Autodesk Inventor part; units mm, degrees
ref_plane "YZ Plane" through (0, 0, 0) normal (1, 0, 0) x (0, 1, 0)
ref_plane "XZ Plane" through (0, 0, 0) normal (0, 1, 0) x (-1, 0, 0)
ref_plane "XY Plane" through (0, 0, 0) normal (0, 0, 1) x (1, 0, 0)
sketch "Sketch1" plane through (0, 0, 0) normal (0, 0, 1) x (1, 0, 0)
  line L0 (0, 37.7) -> (0, -2.9)
  line L1 (-79.8, 0) -> (106.4, 0)
  line L2 (-66.5, 0) -> (66.5, 0)
  line L3 (66.5, 0) -> (66.5, 29)
  line L4 (66.5, 29) -> (-66.5, 29)
  line L5 (-66.5, 29) -> (-66.5, 0)
  dimension "d0" = 133
  dimension "d1" = 29
extrude "Extrusion1" add sketch "Sketch1" along normal blind 1
decal "Decal1"
decal "Decal2"
sketch "Sketch5" plane through (0, 0, 1) normal (0, 0, 1) x (1, 0, 0)
  line L0 (-66.5, 0) -> (-66.5, 29)
  line L1 (66.5, 29) -> (66.5, 0)
  line L2 (-66.5, 19.147) -> (-65.5825, 19.147)
  line L3 (-65.5825, 19.147) -> (-65.5825, 15.2864)
  line L4 (-65.5825, 15.2864) -> (-66.5, 15.2864)
  line L5 (-66.5, 15.2864) -> (-66.5, 19.147)
  line L6 (-66.5, 11.2859) -> (-65.5825, 11.2859)
  line L7 (-65.5825, 11.2859) -> (-65.5825, 7.4252)
  line L8 (-65.5825, 7.4252) -> (-66.5, 7.4252)
  line L9 (-66.5, 7.4252) -> (-66.5, 11.2859)
  circle A0 centre (-65.5825, 17.2167) radius 1.9303
  circle A1 centre (-65.5825, 9.3555) radius 1.9303
  line L10 (66.5, 19.4238) -> (65.1393, 19.4238)
  line L11 (65.1393, 19.4238) -> (65.1393, 15.6247)
  line L12 (65.1393, 15.6247) -> (66.5, 15.6247)
  line L13 (66.5, 15.6247) -> (66.5, 19.4238)
  line L14 (66.5, 11.6256) -> (65.3393, 11.6256)
  line L15 (65.3393, 11.6256) -> (65.3393, 7.8264)
  line L16 (65.3393, 7.8264) -> (66.5, 7.8264)
  line L17 (66.5, 7.8264) -> (66.5, 11.6256)
  circle A2 centre (65.1393, 17.5243) radius 1.8996
  circle A3 centre (65.3393, 9.726) radius 1.8996
  circle A4 centre (-64.4646, 1.8448) radius 1.5
  circle A5 centre (64.8231, 1.8448) radius 1.5
  dimension "d12" = 3
extrude "Extrusion2" cut sketch "Sketch5" against normal through all
sketch "Sketch6" plane through (0, 0, 1) normal (0, 0, 1) x (1, 0, 0)
  line L0 (66.5, 0) -> (-66.5, 0)
  line L1 (3.433, 2.75) -> (4.933, 2.75)
  line L2 (4.933, 2.75) -> (4.933, 0)
  line L3 (4.933, 0) -> (3.433, 0)
  line L4 (3.433, 0) -> (3.433, 2.75)
  circle A0 centre (4.183, 2.75) radius 0.75
  dimension "d15" = 1.5
  dimension "d16" = 2.75
extrude "Extrusion3" cut sketch "Sketch6" against normal through all
sketch "Sketch7" plane through (0, 0, 1) normal (0, 0, 1) x (1, 0, 0)
  line L0 (-46.1031, 8.3659) -> (-58.1031, 8.3659)
  line L1 (-58.1031, 8.3659) -> (-58.1031, 22.3659)
  line L2 (-58.1031, 22.3659) -> (-46.1031, 22.3659)
  line L3 (-46.1031, 22.3659) -> (-46.1031, 8.3659)
  line L4 (-36.7296, 22.3659) -> (-24.7296, 22.3659)
  line L5 (-24.7296, 22.3659) -> (-24.7296, 8.3659)
  line L6 (-24.7296, 8.3659) -> (-36.7296, 8.3659)
  line L7 (-36.7296, 8.3659) -> (-36.7296, 22.3659)
  line L8 (22.9991, 22.3659) -> (34.9991, 22.3659)
  line L9 (34.9991, 22.3659) -> (34.9991, 8.3659)
  line L10 (34.9991, 8.3659) -> (22.9991, 8.3659)
  line L11 (22.9991, 8.3659) -> (22.9991, 22.3659)
  line L12 (40.9859, 22.3659) -> (52.9859, 22.3659)
  line L13 (52.9859, 22.3659) -> (52.9859, 8.3659)
  line L14 (52.9859, 8.3659) -> (40.9859, 8.3659)
  line L15 (40.9859, 8.3659) -> (40.9859, 22.3659)
  dimension "d21" = 14
  dimension "d22" = 12
extrude "Extrusion4" add sketch "Sketch7" along normal blind 0.5
sketch "Sketch8" plane through (0, 0, 0) normal (0, 0, -1) x (-1, 0, 0)
  line L0 (-58.0858, 22.4822) -> (-46.5858, 22.4822)
  line L1 (-46.5858, 22.4822) -> (-46.5858, 8.4822)
  line L2 (-46.5858, 8.4822) -> (-58.0858, 8.4822)
  line L3 (-58.0858, 8.4822) -> (-58.0858, 22.4822)
  line L4 (-36.8395, 22.4822) -> (-25.3395, 22.4822)
  line L5 (-25.3395, 22.4822) -> (-25.3395, 8.4822)
  line L6 (-25.3395, 8.4822) -> (-36.8395, 8.4822)
  line L7 (-36.8395, 8.4822) -> (-36.8395, 22.4822)
  line L8 (23.4032, 22.2455) -> (34.9032, 22.2455)
  line L9 (34.9032, 22.2455) -> (34.9032, 8.4822)
  line L10 (34.9032, 8.4822) -> (23.4032, 8.4822)
  line L11 (23.4032, 8.4822) -> (23.4032, 22.2455)
  line L12 (41.476, 22.1379) -> (52.976, 22.1379)
  line L13 (52.976, 22.1379) -> (52.976, 8.4822)
  line L14 (52.976, 8.4822) -> (41.476, 8.4822)
  line L15 (41.476, 8.4822) -> (41.476, 22.1379)
  dimension "d28" = 11.5
  dimension "d29" = 14
extrude "Extrusion5" add sketch "Sketch8" along normal blind 0.5
sketch "Sketch3" plane through (0, 0, 1) normal (0, 0, 1) x (1, 0, 0)
  line L0 (-66.5, 29) -> (66.5, 29) construction
  line L1 (66.5, 29) -> (66.5, -0.391) construction
  line L2 (66.5, -0.391) -> (-66.5, -0.391) construction
  line L3 (-66.5, -0.391) -> (-66.5, 29) construction
sketch "Sketch4" plane through (0, 0, 0) normal (0, 0, -1) x (-1, 0, 0)
  line L0 (-66.5, 29) -> (66.5, 29) construction
  line L1 (66.5, 29) -> (66.5, -0.391) construction
  line L2 (66.5, -0.391) -> (-66.5, -0.391) construction
  line L3 (-66.5, -0.391) -> (-66.5, 29) construction
properties part number "config - ram"
The listing builds one solid part. Answer for the finished solid, in the listing's coordinates (mm). Coordinates: 2 decimals unless noted, no trailing zeros. Loops run counter-clockwise (first coordinate to the right, second up) from the corner with the lowest first, then second, coordinate; pieces in that order, holes last. Notation, with made-up numbers: M 41.5,70.5 L 66.5,70.5 A24 ccw 66.5,81.5 Z; hole C 51.25,-23 d7. An arc over 180 degrees is marked long. Answer in a Markdown table with one row per item.
1) Find the intervals of material crossed by probe 1 along X at (y, z) = (10.75, 1.2); probe 2 along X at (y, z) = (17.5, -0.1); probe 3 along Y at (x, z) = (28, 1.2), in increasing order.
Answers below:
| item | result |
|---|---|
| probe 1 | -58.1 to -46.1, -36.73 to -24.73, 23 to 35, 40.99 to 52.99 |
| probe 2 | -52.98 to -41.48, -34.9 to -23.4, 25.34 to 36.84, 46.59 to 58.09 |
| probe 3 | 8.37 to 22.37 |
2) Determine the mould class of faces 1 (the cylindrical face through (63.325, 1.911, 0.507)), 2 (the flat face through (-47, 15, -0.5)) for opening direction X: released by +X, released by -X, zero draft, split by the parting line, or undercut.
Answers below:
| item | result |
|---|---|
| face 1 | undercut |
| face 2 | zero draft |
3) Given pin 1 (12 mm diameter, centred on x = 5.5, y = 13.5, fed in from +Z); pin 2 (1 mm diameter, centred on y = 8, z = 0, fed in from +X); pin 3 (0.6 mm diameter, centred on y = 15.5, z = 1.5, fed in from +X); pin 4 (0.6 mm diameter, centred on y = 16.5, z = 1, fed in from +X), each flat-ended and moving along its own axis, determine where each tip first touches the part or whether it passes through.
Answers below:
| item | result |
|---|---|
| pin 1 | z = 1 |
| pin 2 | x = 66.5 |
| pin 3 | x = 52.99 |
| pin 4 | x = 63.78 |
4) Find section C-C (y = 6). Determine the outline of the cut face in (x, z).
Answers below:
| item | result |
|---|---|
| outline | M -66.5,0 L 66.5,0 L 66.5,1 L -66.5,1 Z |
5) Find section B-B (z = 0.6). Determine the outline of the cut face in (x, y), then the cut area to 3 significant figures.
Answers below:
| item | result |
|---|---|
| outline | M -66.5,0 L 3.43,0 L 3.43,2.75 A0.75 cw 4.93,2.75 L 4.93,0 L 66.5,0 L 66.5,7.83 L 65.34,7.83 A1.9 cw 65.34,11.63 L 66.5,11.63 L 66.5,15.62 L 65.14,15.62 A1.9 cw 65.14,19.42 L 66.5,19.42 L 66.5,29 L -66.5,29 L -66.5,19.15 L -65.58,19.15 A1.93 cw -65.58,15.29 L -66.5,15.29 L -66.5,11.29 L -65.58,11.29 A1.93 cw -65.58,7.43 L -66.5,7.43 Z; hole C -64.46,1.84 d3; hole C 64.82,1.84 d3 |
| area | 3,800 mm^2 |
6) Find section A-A (x = -33.5). Determine the outline of the cut face in (y, z), then the cut area to 3 significant figures.
Answers below:
| item | result |
|---|---|
| outline | M 0,0 L 8.48,0 L 8.48,-0.5 L 22.25,-0.5 L 22.25,0 L 29,0 L 29,1 L 22.37,1 L 22.37,1.5 L 8.37,1.5 L 8.37,1 L 0,1 Z |
| area | 42.9 mm^2 |
7) Find section D-D (x = 43.5). Determine the outline of the cut face in (y, z).
Answers below:
| item | result |
|---|---|
| outline | M 0,0 L 29,0 L 29,1 L 22.37,1 L 22.37,1.5 L 8.37,1.5 L 8.37,1 L 0,1 Z |
